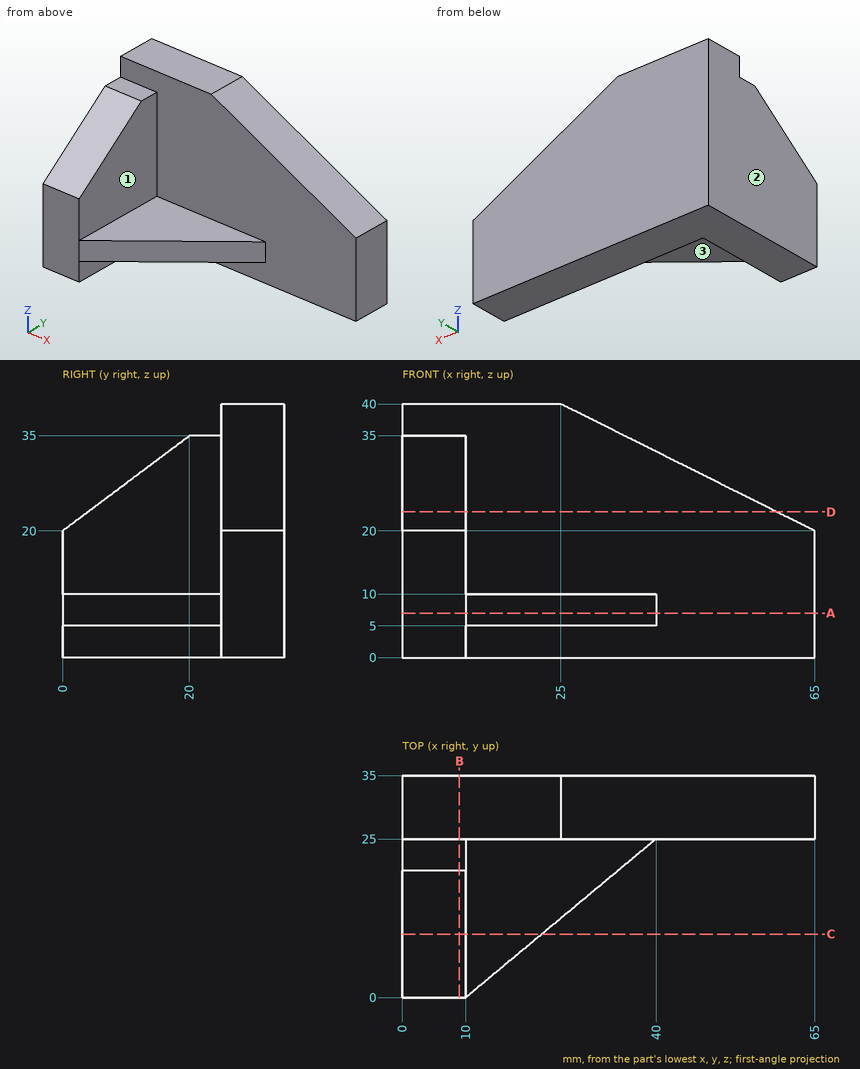
Here's the drawing with two shaded views (mm, measured from the low corner). I have some questions. A direction names the side the tool comes from. Coordinates: 2 decimals unless noted, no trailing zeros. Loops run counter-clockwise (first coordinate to the right, second up) from the corner with the lowest first, then second, coordinate; pieces in that order, holes last. Notation, with made-up numbers: M 46.5,0 L 62.5,0 A13 cw 62.5,21 Z; hole C 28,-10.5 d11. An arc over 180 degrees is marked long. Return JSON: item names as keys, results as strings. Group by question number.
Item 1: If I drill on L1, parallel to X at y = 17.5, z = 24.5; L2, parallel to Y at x = 21.5, z = 4; L3, parallel to Z at x = 24, y = 22.5, over which ranges is the centre line in solid material (lowest first)? Write a range as from..to.
Item 2: Imagine slicing it at B-B (x = 9). Please give me the cut outline in (y, z).
Item 3: Imagine slicing it at A-A (z = 7). Please give me the cut outline in (x, y), and give its area (4 significant figures).
Item 4: Imagine slicing it at C-C (y = 10). Please give me the cut outline in (x, z).
Item 5: Imagine slicing it at D-D (z = 23). Please give me the cut outline in (x, y).
Item 6: I'm going to push flat-ended pins straight in: pin 1 Ø7.5 at (x, y) = (32.5, 15.5) entering from +Z; pin 2 Ø2.5 at (y, z) = (18, 2.5) entering from +X; pin 3 Ø4 at (x, y) = (6, 23.5) entering from +Z; pin 4 Ø10 at (x, z) = (33, 7) entering from -Y. Where does each tip first touch, or does it pass through?
Item 7: On a 3-axis mill with a long thin cutter (end or side, diameter ignored), from which of +Z, -Z, +X, -X, +Y, -Y can I reach the whole of each face in a straight line? I mean the marked faces 1, 2 and 3. Say none if no direction works.
Verdict:
{
 "1": {"L1": "x = 0..10", "L2": "y = 25..35", "L3": "z = 5..10"},
 "2": {"outline": "M 0,0 L 35,0 L 35,40 L 25,40 L 25,35 L 20,35 L 0,20 Z"},
 "3": {"outline": "M 0,0 L 10,0 L 40,25 L 65,25 L 65,35 L 0,35 Z", "area": "1,275 mm^2"},
 "4": {"outline": "M 0,0 L 10,0 L 10,5 L 22,5 L 22,10 L 10,10 L 10,27.5 L 0,27.5 Z"},
 "5": {"outline": "M 0,4 L 10,4 L 10,25 L 59,25 L 59,35 L 0,35 Z"},
 "6": {"pin 1": "stops at z = 10", "pin 2": "stops at x = 10", "pin 3": "stops at z = 40", "pin 4": "stops at y = 15"},
 "7": {"face 1": "+Z, +X, -Y", "face 2": "+Z, -Z, -X, +Y, -Y", "face 3": "-Z, +X, -Y"}
}
